from build123d import *

# Parameters (mm, degrees)
F0_W     = 300
F0_H     = 200
F1_DEPTH = 250
F2_T     = -25
F4_D     = 50


with BuildPart() as f1:
    # F0 (on Top) → F1 (new body)
    with BuildSketch(Plane.XY):
        Rectangle(F0_W, F0_H)
    extrude(amount=F1_DEPTH)

    # F2
    f2_openings = [f1.faces().sort_by_distance(p)[0] for p in [
        (0, 0, 0),
    ]]
    offset(amount=F2_T, openings=f2_openings)

    # F4 (through all)
    with Locations(Plane.XY.offset(250)):
        with Locations((79.174198, 31.202247)):
            Hole(F4_D / 2)


solid = f1.part
Verification items for the finished model (mm, model axes). A direction names the side the tool comes from. Round coordinates to 2 decimals unless told otherwise and drop trailing zeros. Loops run counter-clockwise (first coordinate to the right, second up) from the corner with the lowest first, then second, coordinate; pieces in that order, holes last. Notation, with made-up numbers: (79, 7) - (92, 7) arc R26 cw to (92, 24) - close; hole circle Ø7 at (7.5, -21). An arc over 180 degrees is marked (long way). Write item = value, one per line.
Q1. Sectioned sample at A-A on z = 76. Record the boundary of the cut face in (x, y).
Here are the results:
outline = (-150, -100) - (150, -100) - (150, 100) - (-150, 100) - close; hole (-125, -75) - (125, -75) - (125, 75) - (-125, 75) - close
Q2. Sectioned sample at B-B on y = 22.5. Record the boundary of the cut face in (x, z), plus the area to 3 significant figures.
Here are the results:
outline = (-150, 0) - (-125, 0) - (-125, 225) - (55.74, 225) - (55.74, 250) - (-150, 250) - close; (102.61, 225) - (125, 225) - (125, 0) - (150, 0) - (150, 250) - (102.61, 250) - close
area = 17,600 mm^2
Q3. Material ranges on L1, parallel to X at y = 17.5, z = 136; L2, parallel to Y at x = -79.5, z = 163.5; L3, parallel to Z at x = -49, y = 12.5, recorded low to high.
Here are the results:
L1 = -150 to -125, 125 to 150
L2 = -100 to -75, 75 to 100
L3 = 225 to 250
Q4. Tool access check on faces 1 (the flat face through (-2, 1, 225)), 2 (the flat face through (-2, -100, 123)). Record the directions out of +Z, -Z, +X, -X, +Y, -Y that give a thin tool (end or side, any length) a straight path to the whole face; none if there is none.
Here are the results:
face_1 = -Z
face_2 = +Z, -Z, +X, -X, -Y
Q5. Sectioned sample at C-C on x = 98.5. Record the boundary of the cut face in (y, z), plus the area to 3 significant figures.
Here are the results:
outline = (-100, 0) - (-75, 0) - (-75, 225) - (15.34, 225) - (15.34, 250) - (-100, 250) - close; (47.06, 225) - (75, 225) - (75, 0) - (100, 0) - (100, 250) - (47.06, 250) - close
area = 15,500 mm^2
Q6. Depth check by flat-ended pin: pin 1 (3 mm diameter, centred on x = -37, y = -51, fed in from -Z). Enter the tip coordinate at first touch or a pass-through.
Here are the results:
pin_1 = 225
Q7. Mould release check, pull along X, two halves, no side actions. Record for faces 3 (the flat face through (-150, -1, 123)), 4 (the flat face through (-2, -75, 111)), 5 (the flat face through (-2, -87, 0)): +X half, -X half, draft (parallel to the pull), parting line (faces both ways), or undercut.
Here are the results:
face_3 = -X half
face_4 = undercut
face_5 = draft
Q8. Sectioned sample at D-D on y = -36. Record the boundary of the cut face in (x, z).
Here are the results:
outline = (-150, 0) - (-125, 0) - (-125, 225) - (125, 225) - (125, 0) - (150, 0) - (150, 250) - (-150, 250) - close
